from build123d import *

# Parameters (mm, degrees)
F1_DEPTH = 60
F2_T     = -2
F3_W     = 52
F3_H     = 116
F4_DEPTH = 35


with BuildPart() as f1:
    # F0 (on Top) → F1 (new body, symmetric)
    with BuildSketch(Plane.XY):
        with BuildLine():
            Line((-30, 0), (30, 0))
            ThreePointArc((30, 0), (0, 30), (-30, 0))
        make_face()
    extrude(amount=F1_DEPTH, both=True)

    # F2
    f2_openings = [f1.faces().sort_by_distance(p)[0] for p in [
        (0, 0, 0),
    ]]
    offset(amount=F2_T, openings=f2_openings)

    # F3 (on Front) → F4 (cut)
    with BuildSketch(Plane.XZ):
        Rectangle(F3_W, F3_H)
    extrude(amount=-F4_DEPTH, mode=Mode.SUBTRACT)


solid = f1.part
Design review of the part built by this model. Coordinates are the model's own, in mm. A direction names the side the tool comes from. Round coordinates to 2 decimals unless told otherwise and drop trailing zeros. Write each loop counter-clockwise with the first axis right and the second up, starting at its lowest first coordinate (ties: lowest second). Pieces come first, ordered by that corner, then holes. Notation, with made-up numbers: (-28, 60.5) -> (14, 60.5) arc R30 cw to (14, 95.5) -> close; hole circle Ø9 at (43.5, 39.5). An arc over 180 degrees is marked (long way). One line per question, with ' | ' between items.
(1) Machinability: for faces 4 (the flat face through (0, 12, -60)), 5 (the flat face through (26, 13, -1)), 6 (the cylindrical face through (27.51, 5.22, 0.81)), which of the approach directions +Z, -Z, +X, -X, +Y, -Y give a long, thin tool a straight path to every point of the face, cutting with its end or side? Answer none if there is none.
Result sheet:
face 4: -Z, +X, -X, +Y, -Y | face 5: +Y, -Y | face 6: -Y
(2) Draft analysis for pull direction Z (two halves, no side actions). For faces 1 (the flat face through (0, 12, 58)), 2 (the flat face through (0, 12, 60)), 3 (the flat face through (-29, 0, 18)), state which applies: released by +Z, released by -Z, zero draft, split by the parting line, or undercut.
Result sheet:
face 1: undercut | face 2: released by +Z | face 3: zero draft
(3) Insertion check: P1, Ø4, axis at y = 7, z = 28.5, coming from the +X side; P2, Ø3.5, axis at y = 12.5, z = 9, coming from the +X side; P3, Ø1, axis at y = 9, z = 19.5, coming from the +X side. Each pin has a flat end and moves straight along its axis. Give the tip position at first contact, or say it passes through.
Result sheet:
P1: x = 29.58 | P2: x = 28.01 | P3: x = 28.77
(4) Wall thickness on line 1 (Z direction, x = -15, y = 21); line 2 (X direction, y = 9, z = -11.5); line 3 (X direction, y = 8.75, z = 52): over which ranges is each line inside the solid? List them lowest first. Write a range as [from, to].
Result sheet:
line 1: [-60, -58], [58, 60] | line 2: [-28.62, -26.51], [26.51, 28.62] | line 3: [-28.7, -26.6], [26.6, 28.7]
(5) Take a section at A-A, the plane x = 0. State the section outline as (y, z) points.
Result sheet:
outline: (0, -60) -> (30, -60) -> (30, -58) -> (0, -58) -> close; (0, 58) -> (30, 58) -> (30, 60) -> (0, 60) -> close
(6) Take a section at B-B, the plane z = 36.5. State the section outline as (x, y) points, and give its area (3 significant figures).
Result sheet:
outline: (-30, 0) -> (-28, 0) arc R28 cw to (-26, 10.39) -> (-26, 14.97) arc R30 ccw to start; (26, 10.39) arc R28 cw to (28, 0) -> (30, 0) arc R30 ccw to (26, 14.97) -> close | area: 53.0 mm2
